Check sheet for the modelled part. Datum: model origin and axes. Units: mm. A direction names the side the tool comes from. Coordinates: 2 decimals unless noted, no trailing zeros. Write each loop counter-clockwise with the first axis right and the second up, starting at its lowest first coordinate (ties: lowest second). Pieces come first, ordered by that corner, then holes. Notation, with made-up numbers: (56, -9) - (61, -9) arc R19 ccw to (61, 27) - close; hole circle Ø5 at (35, 44). An arc over 180 degrees is marked (long way). Write each question's results on one line, items separated by ' | '.
from build123d import *

# Parameters (mm, degrees)
SKETCH1_W           = 19.05
SKETCH1_H           = 38.1
SKETCH1_W_2         = 12.7
SKETCH1_H_2         = 31.75
BOSS_EXTRUDE1_DEPTH = 127
SKETCH2_R           = 3.175
CUT_EXTRUDE1_DEPTH  = 20.05
CUT_EXTRUDE2_REACH  = 21.05
SKETCH3_R           = 4.7625
SKETCH4_R           = 1.5875
UCHAN_MOUNT_DEPTH   = 20.05
CUT_EXTRUDE4_REACH  = 21.05
SKETCH5_R           = 4.7625
CUT_EXTRUDE5_DEPTH  = 2.54


with BuildPart() as part:
    # Sketch1 → Boss-Extrude1 (new body)
    with BuildSketch(Plane(origin=(0, 0, 0), x_dir=(1, 0, 0), z_dir=(0, 1, 0))):
        with Locations((9.525, 19.05)):
            Rectangle(SKETCH1_W, SKETCH1_H)
        with Locations((9.525, 19.05)):
            Rectangle(SKETCH1_W_2, SKETCH1_H_2, mode=Mode.SUBTRACT)
    extrude(amount=BOSS_EXTRUDE1_DEPTH)

    # Sketch2 → Cut-Extrude1 (cut, through all)
    with BuildSketch(Plane(origin=(19.05, 0, 0), x_dir=(0, 0, -1), z_dir=(1, 0, 0))):
        with Locations((19.05, 12.7)):
            Circle(SKETCH2_R)
        with Locations((19.05, 32.69996)):
            Circle(SKETCH2_R)
        with Locations((19.05, 94.30004)):
            Circle(SKETCH2_R)
        with Locations((19.05, 114.3)):
            Circle(SKETCH2_R)
    extrude(amount=-CUT_EXTRUDE1_DEPTH, mode=Mode.SUBTRACT)

    # Sketch3 → Cut-Extrude2 (cut, up to next)
    with BuildSketch(Plane(origin=(19.05, 0, 0), x_dir=(0, 0, -1), z_dir=(1, 0, 0)), mode=Mode.PRIVATE) as cut_extrude2_sk1:
        with Locations((19.05, 114.3)):
            Circle(SKETCH3_R)
    cut_extrude2_tool1 = extrude(cut_extrude2_sk1.sketch, amount=-CUT_EXTRUDE2_REACH, mode=Mode.PRIVATE) & part.part
    add(cut_extrude2_tool1.solids().sort_by_distance((19.05, 114.3, -19.05))[0], mode=Mode.SUBTRACT)
    # Sketch3 → Cut-Extrude2 (cut, up to next)
    with BuildSketch(Plane(origin=(19.05, 0, 0), x_dir=(0, 0, -1), z_dir=(1, 0, 0)), mode=Mode.PRIVATE) as cut_extrude2_sk2:
        with Locations((19.05, 94.30004)):
            Circle(SKETCH3_R)
    cut_extrude2_tool2 = extrude(cut_extrude2_sk2.sketch, amount=-CUT_EXTRUDE2_REACH, mode=Mode.PRIVATE) & part.part
    add(cut_extrude2_tool2.solids().sort_by_distance((19.05, 94.30004, -19.05))[0], mode=Mode.SUBTRACT)
    # Sketch3 → Cut-Extrude2 (cut, up to next)
    with BuildSketch(Plane(origin=(19.05, 0, 0), x_dir=(0, 0, -1), z_dir=(1, 0, 0)), mode=Mode.PRIVATE) as cut_extrude2_sk3:
        with Locations((19.05, 32.69996)):
            Circle(SKETCH3_R)
    cut_extrude2_tool3 = extrude(cut_extrude2_sk3.sketch, amount=-CUT_EXTRUDE2_REACH, mode=Mode.PRIVATE) & part.part
    add(cut_extrude2_tool3.solids().sort_by_distance((19.05, 32.69996, -19.05))[0], mode=Mode.SUBTRACT)
    # Sketch3 → Cut-Extrude2 (cut, up to next)
    with BuildSketch(Plane(origin=(19.05, 0, 0), x_dir=(0, 0, -1), z_dir=(1, 0, 0)), mode=Mode.PRIVATE) as cut_extrude2_sk4:
        with Locations((19.05, 12.7)):
            Circle(SKETCH3_R)
    cut_extrude2_tool4 = extrude(cut_extrude2_sk4.sketch, amount=-CUT_EXTRUDE2_REACH, mode=Mode.PRIVATE) & part.part
    add(cut_extrude2_tool4.solids().sort_by_distance((19.05, 12.7, -19.05))[0], mode=Mode.SUBTRACT)

    # Sketch4 → UChan_Mount (cut, through all)
    with BuildSketch(Plane(origin=(19.05, 0, 0), x_dir=(0, 0, -1), z_dir=(1, 0, 0))):
        with Locations((19.05, 22.69998)):
            Circle(SKETCH4_R)
        with Locations((19.05, 63.5)):
            Circle(SKETCH4_R)
        with Locations((19.05, 104.30002)):
            Circle(SKETCH4_R)
    extrude(amount=-UCHAN_MOUNT_DEPTH, mode=Mode.SUBTRACT)

    # Sketch5 → Cut-Extrude4 (cut, up to next)
    with BuildSketch(Plane.ZY, mode=Mode.PRIVATE) as cut_extrude4_sk1:
        with Locations((-19.05, 104.30002)):
            Circle(SKETCH5_R)
    cut_extrude4_tool1 = extrude(cut_extrude4_sk1.sketch, amount=-CUT_EXTRUDE4_REACH, mode=Mode.PRIVATE) & part.part
    add(cut_extrude4_tool1.solids().sort_by_distance((0, 104.30002, -19.05))[0], mode=Mode.SUBTRACT)
    # Sketch5 → Cut-Extrude4 (cut, up to next)
    with BuildSketch(Plane.ZY, mode=Mode.PRIVATE) as cut_extrude4_sk2:
        with Locations((-19.05, 63.5)):
            Circle(SKETCH5_R)
    cut_extrude4_tool2 = extrude(cut_extrude4_sk2.sketch, amount=-CUT_EXTRUDE4_REACH, mode=Mode.PRIVATE) & part.part
    add(cut_extrude4_tool2.solids().sort_by_distance((0, 63.5, -19.05))[0], mode=Mode.SUBTRACT)
    # Sketch5 → Cut-Extrude4 (cut, up to next)
    with BuildSketch(Plane.ZY, mode=Mode.PRIVATE) as cut_extrude4_sk3:
        with Locations((-19.05, 22.69998)):
            Circle(SKETCH5_R)
    cut_extrude4_tool3 = extrude(cut_extrude4_sk3.sketch, amount=-CUT_EXTRUDE4_REACH, mode=Mode.PRIVATE) & part.part
    add(cut_extrude4_tool3.solids().sort_by_distance((0, 22.69998, -19.05))[0], mode=Mode.SUBTRACT)

    # Sketch6 → Cut-Extrude5 (cut)
    with BuildSketch(Plane(origin=(19.05, 0, 0), x_dir=(0, 0, -1), z_dir=(1, 0, 0))):
        Polygon((0, 127), (6.5373666, 127), (0, 122.48760451), align=None)
    extrude(amount=-CUT_EXTRUDE5_DEPTH, mode=Mode.SUBTRACT)


solid = part.part
1. Sectioned sample at C-C (x = 5.75). Record the cut outline in (y, z) (3 decimals), then the cut area to 3 significant figures.
Values follow:
outline: (0, -38.1) - (127, -38.1) - (127, -34.925) - (0, -34.925) - close; (0, -3.175) - (127, -3.175) - (127, 0) - (0, 0) - close | area: 806 mm^2
2. Sectioned sample at D-D (z = -19.05). Give the number of separate pieces and of enclosed holes in the cut face, then the cut area to 3 significant figures.
Values follow:
separate pieces: 16 | enclosed holes: 0 | area: 484 mm^2
3. Access from +Z, -Z, +X, -X, +Y, -Y to the whole of each face (thin tool, end or side, straight path). Record for faces 1 (the flat face through (9, 63, -34.925)), 2 (the cylindrical face through (17.48, 119.02, -18.43)), 3 (the flat face through (17.798, 124.775, -3.314)).
Values follow:
face 1: +Y, -Y | face 2: +X | face 3: +Z, +X, +Y
4. Sectioned sample at B-B (z = -12). Record the cut outline in (x, y) (3 decimals), then the cut area to 3 significant figures.
Values follow:
outline: (0, 0) - (3.175, 0) - (3.175, 127) - (0, 127) - close; (15.875, 0) - (19.05, 0) - (19.05, 127) - (15.875, 127) - close | area: 806 mm^2
5. Draft check along Z on faces 4 (the cylindrical face through (1.61, 97.45, -18.64)), 5 (the flat face through (0, 63, -10)), 6 (the flat face through (9, 63, 0)). Enter one of: pulls with the +Z half, pulls with the -Z half, needs draft (parallel to the pull), parting line crosses it, or undercut.
Values follow:
face 4: undercut | face 5: needs draft | face 6: pulls with the +Z half
6. Material ranges on L1, parallel to Z at x = 13.5, y = 59.5 (3 decimals); L2, parallel to X at y = 102.5, z = -8 (3 decimals); L3, parallel to X at y = 101.5, z = -21 (3 decimals), recorded low to high. Write a range as [from, to].
Values follow:
L1: z = [-38.1, -34.925], [-3.175, 0] | L2: x = [0, 3.175], [15.875, 19.05] | L3: x = [15.875, 19.05]
7. Go/stop test with flat-tipped pins: pin 1 (5.5 mm diameter, centred on y = 94.3, z = -19.05, fed in from -X); pin 2 (5.5 mm diameter, centred on y = 22.7, z = -19.05, fed in from -X) (3 decimals). Record where each tip stops, or that it passes through.
Values follow:
pin 1: passes through | pin 2: stops at x = 15.875
